from build123d import *


with BuildPart() as part:
    # 草图1 → 旋转-薄壁3 (revolve)
    with BuildSketch(Plane.XY, mode=Mode.PRIVATE) as revolve_3_sk:
        with BuildLine():
            Line((-1, -33.401673559), (-25.4, -33.401673559))
            Line((-25.4, -33.401673559), (-25.4, -28.401673559))
            Line((-25.4, -28.401673559), (-15.4, -18.4))
            ThreePointArc((-15.4, -18.4), (-25, 0.8), (-15.4, 20))
            Line((-15.4, 20), (-25, 30.001673559))
            Line((-25, 30.001673559), (-25, 35.001673559))
            Line((-25, 35.001673559), (-1, 35.001673559))
            Line((-1, 35.001673559), (-1, 36.001673559))
            Line((-1, 36.001673559), (-26, 36.001673559))
            Line((-26, 36.001673559), (-26, 29.599411836))
            Line((-26, 29.599411836), (-16.885830121, 20.103896015))
            ThreePointArc((-16.885830121, 20.103896015), (-25.999997392, 0.811418377), (-16.903457024, -18.489376731))
            Line((-16.903457024, -18.489376731), (-26.4, -27.987509009))
            Line((-26.4, -27.987509009), (-26.4, -34.401673559))
            Line((-26.4, -34.401673559), (-1, -34.401673559))
            Line((-1, -34.401673559), (-1, -33.401673559))
        make_face()
    revolve(revolve_3_sk.sketch.rotate(Axis((-1, -999.2, 0), (0, 1, 0)), 270), axis=Axis((-1, -999.2, 0), (0, 1, 0)))


solid = part.part
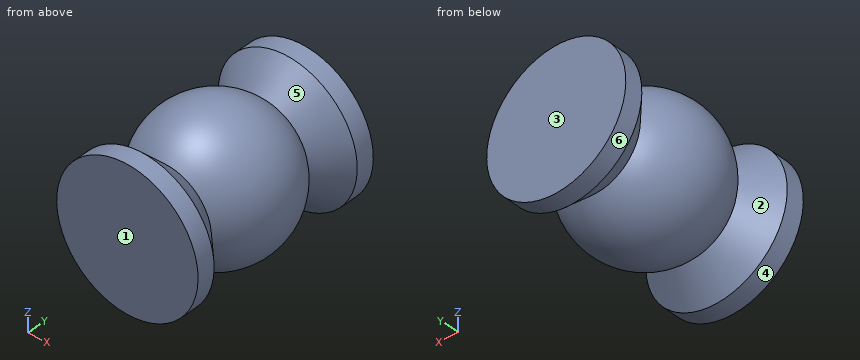
The listing builds one solid part. Answer for the finished solid, in the listing's coordinates (mm). Face numbers are marked on the shaded views. A direction names the side the tool comes from. Round coordinates to 2 decimals unless told otherwise and drop trailing zeros. Write each loop counter-clockwise with the first axis right and the second up, starting at its lowest first coordinate (ties: lowest second). Pieces come first, ordered by that corner, then holes. Notation, with made-up numbers: M 43.5,48 L 51.5,48 A26 ccw 51.5,75 Z; hole C -25,79.25 d5. An arc over 180 degrees is marked long. Write each question's results on one line, items separated by ' | '. Start each with the question number.
(1) The part is cut by section B-B, the plane x = -17.5. Give the number of separate pieces and of enclosed holes in the cut face, and give its area (3 significant figures).
(2) For the marked faces 4, 5 and 6, determine the directions among +Z, -Z, +X, -X, +Y, -Y from which every point of the face is accessible in a straight line to the end or side of a thin tool.
(3) The part is cut by section A-A, the plane z = 0. Write down the section's boundary in (x, y), and give its area (3 significant figures).
(4) The part is cut by section C-C, the plane x = -1. Write down the section's boundary in (y, z).
(5) Find the intervals of material crossed by line 1 (Y direction, x = 9, z = -2); line 2 (X direction, y = -29.85, z = 0); line 3 (Y direction, x = 17.5, z = -3), in increasing order.
(6) Each of these flat-tipped pins is pushed along its axis until it touches: P1, Ø10, axis at x = -15, y = 5, coming from the +Z side; P2, Ø4, axis at x = -13.5, y = 19.5, coming from the -Z side; P3, Ø10, axis at y = -24.5, z = -9.5, coming from the -X side. Where does it stop, or does it pass through?
(7) Determine the mould class of the marked faces 1, 2 and 3 for opening direction Y: +Y half, -Y half, draft (parallel to the pull), parting line (faces both ways), or undercut.
Worked answers:
1) separate pieces: 3 | enclosed holes: 3 | area: 363 mm²
2) face 4: +Y, -Y | face 5: none | face 6: +Y
3) outline: M -26.4,-34.4 L 24.4,-34.4 L 24.4,-27.99 L 14.9,-18.49 A25 ccw 14.89,20.1 L 24,29.6 L 24,36 L -26,36 L -26,29.6 L -16.89,20.1 A25 ccw -16.9,-18.49 L -26.4,-27.99 Z; hole M -25.4,-33.4 L 23.4,-33.4 L 23.4,-28.4 L 13.4,-18.4 A24 ccw 13.4,20 L 23,30 L 23,35 L -25,35 L -25,30 L -15.4,20 A24 ccw -15.4,-18.4 L -25.4,-28.4 Z | area: 265 mm²
4) outline: M -34.4,-25.4 L -27.99,-25.4 L -18.49,-15.9 A25 ccw 20.1,-15.89 L 29.6,-25 L 36,-25 L 36,25 L 29.6,25 L 20.1,15.89 A25 ccw -18.49,15.9 L -27.99,25.4 L -34.4,25.4 Z; hole M -33.4,-24.4 L -28.4,-24.4 L -18.4,-14.4 A24 ccw 20,-14.4 L 30,-24 L 35,-24 L 35,24 L 30,24 L 20,14.4 A24 ccw -18.4,14.4 L -28.4,24.4 L -33.4,24.4 Z
5) line 1: y = -34.4 to -33.4, 35 to 36 | line 2: x = -26.4 to -25.4, 23.4 to 24.4 | line 3: y = -34.4 to -33.4, -22.74 to -21.33, -15.75 to -14.19, 15.79 to 17.35, 23.08 to 24.52, 35 to 36
6) P1: stops at z = 23.08 | P2: stops at z = -14.32 | P3: stops at x = -25.7
7) face 1: -Y half | face 2: undercut | face 3: +Y half
